from build123d import *

# Parameters (mm, degrees)
SKETCH1_W           = 112.7125
SKETCH1_H           = 96.8375
BOSS_EXTRUDE1_DEPTH = 12.7
CUT_EXTRUDE2_START  = -12.7
SKETCH2_R           = 8.334375
CUT_EXTRUDE2_DEPTH  = 89.077000906
CUT_EXTRUDE4_START  = -12.7
SKETCH3_R           = 11.509375
CUT_EXTRUDE4_DEPTH  = 12.7
CUT_EXTRUDE6_START  = 12.7
SKETCH4_R           = 11.509375
CUT_EXTRUDE6_DEPTH  = 12.7
CUT_EXTRUDE8_START  = 12.7
SKETCH5_R           = 16.6497
CUT_EXTRUDE8_DEPTH  = 2.8194
CUT_EXTRUDE10_START = -12.7
SKETCH6_R           = 3.571875
CUT_EXTRUDE10_DEPTH = 7.9375
CUT_EXTRUDE12_START = 12.7
SKETCH7_R           = 3.175
CUT_EXTRUDE12_DEPTH = 7.9375


with BuildPart() as part:
    # Sketch1 → Boss-Extrude1 (new, symmetric)
    with BuildSketch(Plane(origin=(0, 0, 0), x_dir=(1, 0, 0), z_dir=(0, 1, 0))):
        Rectangle(SKETCH1_W, SKETCH1_H)
    extrude(amount=BOSS_EXTRUDE1_DEPTH, both=True)

    # Sketch2 → Cut-Extrude2 (cut, through all)
    with BuildSketch(Plane(origin=(0, 0, 0), x_dir=(1, 0, 0), z_dir=(0, 1, 0)).offset(CUT_EXTRUDE2_START)):
        with Locations(Location((-40.48125, -32.48025, 0), (0, 0, 270))):
            Circle(SKETCH2_R)
        with Locations(Location((40.54475, -32.48025, 0), (0, 0, 270))):
            Circle(SKETCH2_R)
        with Locations(Location((-40.48125, 32.54375, 0), (0, 0, 270))):
            Circle(SKETCH2_R)
        with Locations(Location((40.54475, 32.54375, 0), (0, 0, 270))):
            Circle(SKETCH2_R)
    extrude(amount=CUT_EXTRUDE2_DEPTH, mode=Mode.SUBTRACT)

    # Sketch3 → Cut-Extrude4 (cut)
    with BuildSketch(Plane(origin=(0, 0, 0), x_dir=(1, 0, 0), z_dir=(0, 1, 0)).offset(CUT_EXTRUDE4_START)):
        with Locations(Location((-27.78125, 0.03175, 0), (0, 0, 270))):
            Circle(SKETCH3_R)
        with Locations(Location((18.19275, 0.03175, 0), (0, 0, 270))):
            Circle(SKETCH3_R)
    extrude(amount=CUT_EXTRUDE4_DEPTH, mode=Mode.SUBTRACT)

    # Sketch4 → Cut-Extrude6 (cut)
    with BuildSketch(Plane(origin=(0, 0, 0), x_dir=(1, 0, 0), z_dir=(0, 1, 0)).offset(CUT_EXTRUDE6_START)):
        with Locations(Location((-18.12925, 0.03175, 0), (0, 0, 270))):
            Circle(SKETCH4_R)
        with Locations(Location((27.84475, 0.03175, 0), (0, 0, 270))):
            Circle(SKETCH4_R)
    extrude(amount=-CUT_EXTRUDE6_DEPTH, mode=Mode.SUBTRACT)

    # Sketch5 → Cut-Extrude8 (cut)
    with BuildSketch(Plane(origin=(0, 0, 0), x_dir=(1, 0, 0), z_dir=(0, 1, 0)).offset(CUT_EXTRUDE8_START)):
        with Locations(Location((-18.12925, 0.03175, 0), (0, 0, 270))):
            Circle(SKETCH5_R)
        with Locations(Location((27.84475, 0.03175, 0), (0, 0, 270))):
            Circle(SKETCH5_R)
    extrude(amount=-CUT_EXTRUDE8_DEPTH, mode=Mode.SUBTRACT)

    # Sketch6 → Cut-Extrude10 (cut)
    with BuildSketch(Plane(origin=(0, 0, 0), x_dir=(1, 0, 0), z_dir=(0, 1, 0)).offset(CUT_EXTRUDE10_START)):
        with Locations(Location((49.18075, 0.03175, 0), (0, 0, 270))):
            Circle(SKETCH6_R)
        with Locations(Location((0.15875, -32.48025, 0), (0, 0, 270))):
            Circle(SKETCH6_R)
    extrude(amount=CUT_EXTRUDE10_DEPTH, mode=Mode.SUBTRACT)

    # Sketch7 → Cut-Extrude12 (cut)
    with BuildSketch(Plane(origin=(0, 0, 0), x_dir=(1, 0, 0), z_dir=(0, 1, 0)).offset(CUT_EXTRUDE12_START)):
        with Locations(Location((-49.11725, 0.03175, 0), (0, 0, 270))):
            Circle(SKETCH7_R)
        with Locations(Location((-0.09525, 32.54375, 0), (0, 0, 270))):
            Circle(SKETCH7_R)
    extrude(amount=-CUT_EXTRUDE12_DEPTH, mode=Mode.SUBTRACT)


solid = part.part
Geometry check sheet. Reference: the model listing, model coordinates, mm. A direction names the side the tool comes from. Round coordinates to 2 decimals unless told otherwise and drop trailing zeros. Loops run counter-clockwise (first coordinate to the right, second up) from the corner with the lowest first, then second, coordinate; pieces in that order, holes last. Notation, with made-up numbers: (9, -36) - (29, -36) arc R10 ccw to (29, -30) - close; hole circle Ø1 at (-11.75, -20). An arc over 180 degrees is marked (long way). One line per question, with ' | ' between items. Start each with the question number.
1. Cross-section at B-B on z = -38.5. Record the cut outline in (x, y).
2. Depth check by flat-ended pin: pin 1 (3.5 mm diameter, centred on x = 0, z = 33, fed in from -Y); pin 2 (13 mm diameter, centred on x = -17, z = 4, fed in from +Y); pin 3 (14 mm diameter, centred on x = -18.13, z = -0.03, fed in from -Y); pin 4 (8 mm diameter, centred on x = -30, z = -1, fed in from -Y). Enter the tip coordinate at first touch or a pass-through.
3. Cross-section at D-D on y = -2.5. Record the cut outline in (x, z).
4. Cross-section at C-C on z = -13. Record the cut outline in (x, y).
5. Tool access check on faces 1 (the face through (-4.09, 11.31, 8.92)), 2 (the face through (-34.85, -0.18, -38.69)), 3 (the face through (-33, 0, 0)). Record the directions out of +Z, -Z, +X, -X, +Y, -Y that give a thin tool (end or side, any length) a straight path to the whole face; none if there is none.
6. Cross-section at A-A on y = 7. State how many separate pieces and enclosed holes the cut face has, then the cut area to 3 significant figures.
7. Scan lines: line 1 (Z direction, x = -34, y = 7); line 2 (Z direction, x = -36.5, y = 6.5); line 3 (X direction, y = 0.5, z = 10.5). Record each from-to range of solid material in increasing order. Write a range as [from, to].
8. Draft check along Z on faces 4 (the face through (-45.97, 8.79, -0.45)), 5 (the face through (0, -4.762, 32)), 6 (the face through (-1, 12.7, -1)). Enter one of: released by +Z, released by -Z, zero draft, split by the parting line, or undercut.
Taken from the geometry:
1) outline: (-56.36, -12.7) - (-46.31, -12.7) - (-46.31, 12.7) - (-56.36, 12.7) - close; (-34.65, -12.7) - (34.72, -12.7) - (34.72, 12.7) - (-34.65, 12.7) - close; (46.37, -12.7) - (56.36, -12.7) - (56.36, 12.7) - (46.37, 12.7) - close
2) pin 1: y = -4.76 | pin 2: y = 0 | pin 3: y = -12.7 | pin 4: y = 0
3) outline: (-56.36, -48.42) - (56.36, -48.42) - (56.36, 48.42) - (-56.36, 48.42) - close; hole circle Ø16.67 at (-40.48, -32.54); hole circle Ø16.67 at (-40.48, 32.48); hole circle Ø23.02 at (-27.78, -0.03); hole circle Ø23.02 at (18.19, -0.03); hole circle Ø16.67 at (40.54, -32.54); hole circle Ø16.67 at (40.54, 32.48)
4) outline: (-56.36, -12.7) - (56.36, -12.7) - (56.36, 12.7) - (38.29, 12.7) - (38.29, 9.88) - (17.4, 9.88) - (17.4, 12.7) - (-7.69, 12.7) - (-7.69, 9.88) - (-28.57, 9.88) - (-28.57, 12.7) - (-56.36, 12.7) - close
5) face 1: +Y | face 2: +Y, -Y | face 3: -Y
6) separate pieces: 1 | enclosed holes: 8 | area: 9,150 mm²
7) line 1: [-48.42, -37.78], [-27.3, 27.24], [37.72, 48.42] | line 2: [-48.42, -39.87], [-25.22, 25.16], [39.8, 48.42] | line 3: [-56.36, -22.77], [-13.49, 23.2], [32.49, 56.36]
8) face 4: undercut | face 5: undercut | face 6: zero draft
